```python
from build123d import *

# Parameters (mm, degrees)
SKETCH1_R           = 7.5
SKETCH1_R_2         = 13
BOSS_EXTRUDE1_DEPTH = 10
SKETCH2_R           = 13
SKETCH2_R_2         = 5
BOSS_EXTRUDE2_DEPTH = 10


with BuildPart() as part:
    # Sketch1 → Boss-Extrude1 (new body)
    with BuildSketch(Plane.XY):
        with BuildLine():
            ThreePointArc((25, 100), (0, 125), (-25, 100))
            Line((-25, 100), (-24.805447471, 96.887159533))
            Line((-24.805447471, 96.887159533), (-12.5, -100))
            ThreePointArc((-12.5, -100), (0, -112.5), (12.5, -100))
            Line((12.5, -100), (24.805447471, 96.887159533))
            Line((24.805447471, 96.887159533), (25, 100))
        make_face()
        with Locations((0, -100)):
            Circle(SKETCH1_R, mode=Mode.SUBTRACT)
        with Locations((0, 100)):
            Circle(SKETCH1_R_2, mode=Mode.SUBTRACT)
    extrude(amount=BOSS_EXTRUDE1_DEPTH)

    # Sketch2 → Boss-Extrude2 (add)
    with BuildSketch(Plane.XY.offset(10)):
        with Locations((0, 100)):
            Circle(SKETCH2_R)
        with Locations((0, 100)):
            Circle(SKETCH2_R_2, mode=Mode.SUBTRACT)
    extrude(amount=-BOSS_EXTRUDE2_DEPTH)


solid = part.part
```
Verification items for the finished model (mm, model axes). Coordinates: 2 decimals unless noted, no trailing zeros. Write each loop counter-clockwise with the first axis right and the second up, starting at its lowest first coordinate (ties: lowest second). Pieces come first, ordered by that corner, then holes. Notation, with made-up numbers: (56, -28) - (88, -28) arc R19 ccw to (88, -6) - close; hole circle Ø2 at (17, 76.5). An arc over 180 degrees is marked (long way). Write item = value, one per line.
Q1. Go/stop test with flat-tipped pins: pin 1 Ø9 at (x, y) = (0, 100) entering from -Z; pin 2 Ø3 at (y, z) = (20, 7) entering from -X; pin 3 Ø1.5 at (y, z) = (-47, 8.5) entering from +X; pin 4 Ø4 at (y, z) = (-2.5, 5) entering from -X. Record where each tip stops, or that it passes through.
Answer:
pin_1 = through
pin_2 = -20.09
pin_3 = 15.86
pin_4 = -18.72
Q2. Cross-section at B-B (z = 5). Enter the section's corners in (x, y), plus the area to 3 significant figures.
Answer:
outline = (-25, 100) - (-12.5, -100) arc R12.5 ccw to (12.5, -100) - (25, 100) arc R25 ccw to start; hole circle Ø15 at (0, -100); hole circle Ø10 at (0, 100)
area = 8,470 mm²
Q3. Cross-section at D-D (y = 1.5). Enter the section's corners in (x, z), plus the area to 3 significant figures.
Answer:
outline = (-18.84, 0) - (18.84, 0) - (18.84, 10) - (-18.84, 10) - close
area = 377 mm²
Q4. Material ranges on L1, parallel to Y at x = 0, z = 3; L2, parallel to Y at x = -4, z = 4.5; L3, parallel to X at y = -56.5, z = 8.5, recorded low to high. Write a range as from..to.
Answer:
L1 = -112.5..-107.5, -92.5..95, 105..125
L2 = -111.84..-106.34, -93.66..97, 103..124.68
L3 = -15.22..15.22
Q5. Cross-section at C-C (y = 67). Enter the section's corners in (x, z), plus the area to 3 significant figures.
Answer:
outline = (-22.94, 0) - (22.94, 0) - (22.94, 10) - (-22.94, 10) - close
area = 459 mm²
Q6. Mould release check, pull along Y, two halves, no side actions. Record for faces 1 (the face through (0, 34, 10)), 2 (the face through (0.55, 124.994, 4.93)), 3 (the face through (-1.63, -107.32, 4.93)): released by +Y, released by -Y, zero draft, split by the parting line, or undercut.
Answer:
face_1 = zero draft
face_2 = released by +Y
face_3 = undercut
Q7. Cross-section at A-A (x = 0). Enter the section's corners in (y, z).
Answer:
outline = (-112.5, 0) - (-107.5, 0) - (-107.5, 10) - (-112.5, 10) - close; (-92.5, 0) - (95, 0) - (95, 10) - (-92.5, 10) - close; (105, 0) - (125, 0) - (125, 10) - (105, 10) - close
